The model under review builds one solid part; all positions refer to its coordinate system, in mm. A direction names the side the tool comes from. Round coordinates to 2 decimals unless told otherwise and drop trailing zeros. Order: outer loops, then holes, each group sorted by start corner. A loop starts at its lowest first (then second) coordinate and runs counter-clockwise, first axis right, second up.
```python
from build123d import *

# Parameters (mm, degrees)
SKETCH1_W           = 59.8
SKETCH1_H           = 77.8
BOSS_EXTRUDE1_DEPTH = 3
SKETCH2_R           = 1.5
CUT_EXTRUDE1_DEPTH  = 50.155060777


with BuildPart() as part:
    # Sketch1 → Boss-Extrude1 (new body)
    with BuildSketch(Plane.XY):
        Rectangle(SKETCH1_W, SKETCH1_H)
    extrude(amount=BOSS_EXTRUDE1_DEPTH)

    # Sketch2 → Cut-Extrude1 (cut, through all)
    with BuildSketch(Plane(origin=(0, 0, 0), x_dir=(-1, 0, 0), z_dir=(0, 0, -1))):
        with Locations((0.15, -27.8)):
            Circle(SKETCH2_R)
        with Locations((0.15, 27.8)):
            Circle(SKETCH2_R)
        with BuildLine():
            Line((0.5, -10.5), (0.5, 10.5))
            ThreePointArc((0.5, 10.5), (-4.5, 15.5), (-9.5, 10.5))
            Line((-9.5, 10.5), (-9.5, -10.5))
            ThreePointArc((-9.5, -10.5), (-4.5, -15.5), (0.5, -10.5))
        make_face()
    extrude(amount=-CUT_EXTRUDE1_DEPTH, mode=Mode.SUBTRACT)


solid = part.part
```
(1) For faces 4 (the flat face through (-0.5, 0, 1)), 5 (the flat face through (29.9, -1, 1)), list the 3-axis set-ups (+Z, -Z, +X, -X, +Y, -Y) from which the entire face can be reached by the end or side of a thin tool; tool diameter is ignored.
Data:
face 4: +Z, -Z
face 5: +Z, -Z, +X, +Y, -Y
(2) Insertion check: pin 1 (2.5 mm diameter, centred on x = -0.15, y = -27.8, fed in from +Z). The pin has a flat end and moves straight along its axis. Give the tip position at first contact, or say it passes through.
Data:
pin 1: passes through
(3) Consider section C-C (z = 2.05). Write out the cut boundary in (x, y), and give its area (3 significant figures).
Data:
outline: (-29.9, -38.9) - (29.9, -38.9) - (29.9, 38.9) - (-29.9, 38.9) - close; hole circle Ø3 at (-0.15, -27.8); hole circle Ø3 at (-0.15, 27.8); hole (-0.5, -10.5) arc R5 ccw to (9.5, -10.5) - (9.5, 10.5) arc R5 ccw to (-0.5, 10.5) - close
area: 4,350 mm2
(4) Consider section B-B (y = -27.8). Write out the cut boundary in (x, z).
Data:
outline: (-29.9, 0) - (-1.65, 0) - (-1.65, 3) - (-29.9, 3) - close; (1.35, 0) - (29.9, 0) - (29.9, 3) - (1.35, 3) - close
(5) Draft analysis for pull direction Y (two halves, no side actions). For faces 1 (the cylindrical face through (0.175, -29.264, 1.479)), 2 (the flat face through (0, 38.9, 1)), 3 (the flat face through (-7, 1, 3)), state which applies: pulls with the +Y half, pulls with the -Y half, needs draft (parallel to the pull), parting line crosses it, or undercut.
Data:
face 1: undercut
face 2: pulls with the +Y half
face 3: needs draft
(6) Consider section A-A (x = 4.5). Write out the cut boundary in (y, z).
Data:
outline: (-38.9, 0) - (-15.5, 0) - (-15.5, 3) - (-38.9, 3) - close; (15.5, 0) - (38.9, 0) - (38.9, 3) - (15.5, 3) - close
(7) To check wall thickness, follow probe 1 along X at (y, z) = (10.5, 2.6); probe 2 along Y at (x, z) = (5.5, 2.65); probe 3 along Y at (x, z) = (6, 0.55). State the ranges of each line that lie inside material, in increasing order.
Data:
probe 1: x = -29.9 to -0.5, 9.5 to 29.9
probe 2: y = -38.9 to -15.4, 15.4 to 38.9
probe 3: y = -38.9 to -15.27, 15.27 to 38.9
